Design review of the part built by this model. Coordinates are the model's own, in mm. Face numbers are marked on the shaded views. A direction names the side the tool comes from. Coordinates: 2 decimals unless noted, no trailing zeros. Write each loop counter-clockwise with the first axis right and the second up, starting at its lowest first coordinate (ties: lowest second). Pieces come first, ordered by that corner, then holes. Notation, with made-up numbers: (44.25, -5.75) - (80.25, -5.75) arc R25 cw to (80.25, 9.25) - close; hole circle Ø6 at (43, -6). An arc over 180 degrees is marked (long way). Answer as a JSON object with one key per item and string values.
```python
from build123d import *

# Parameters (mm, degrees)
BOSS_EXTRUDE1_DEPTH = 2.032


with BuildPart() as part:
    # Sketch1 → Boss-Extrude1 (new body)
    with BuildSketch(Plane.XY):
        Polygon((2.794, 7.39775), (-2.794, 7.39775), (-5.5245, 4.66725), (-5.5245, -4.66725), (5.5245, -4.66725), (5.5245, 4.66725), align=None)
        with BuildLine():
            ThreePointArc((1.75976362, 1.016), (0, -2.032), (-1.75976362, 1.016))
            Line((-1.75976362, 1.016), (1.75976362, 1.016))
        make_face(mode=Mode.SUBTRACT)
    extrude(amount=BOSS_EXTRUDE1_DEPTH)


solid = part.part
```
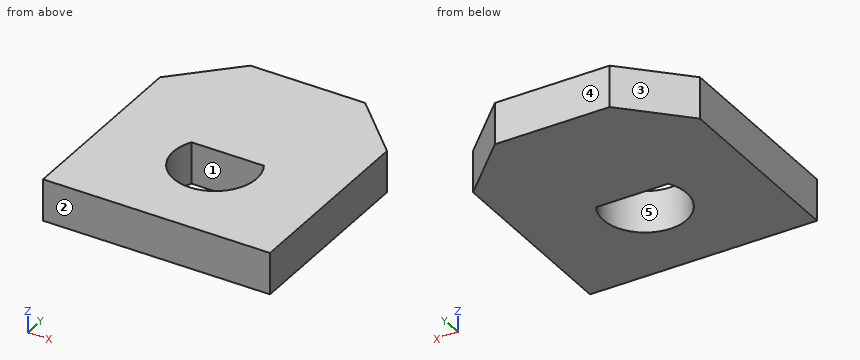
(1) Take a section at D-D, the plane y = 6.25. Write out the cut boundary in (x, z).
Solved:
{"outline": "(-3.94, 0) - (3.94, 0) - (3.94, 2.03) - (-3.94, 2.03) - close"}
(2) Take a section at A-A, the plane z = 1.6. Write out the cut boundary in (x, y).
Solved:
{"outline": "(-5.52, -4.67) - (5.52, -4.67) - (5.52, 4.67) - (2.79, 7.4) - (-2.79, 7.4) - (-5.52, 4.67) - close; hole (-1.76, 1.02) arc R2.03 ccw (long way) to (1.76, 1.02) - close"}
(3) Take a section at B-B, the plane y = 0. Write out the cut boundary in (x, z), and give its area (3 significant figures).
Solved:
{"outline": "(-5.52, 0) - (-2.03, 0) - (-2.03, 2.03) - (-5.52, 2.03) - close; (2.03, 0) - (5.52, 0) - (5.52, 2.03) - (2.03, 2.03) - close", "area": "14.2 mm^2"}
(4) The part is to be moulded in two halves that separate along X. For the marked faces 3, 4 and 5, say which applies: pulls with the +X half, pulls with the -X half, needs draft (parallel to the pull), parting line crosses it, or undercut.
Solved:
{"face 3": "pulls with the -X half", "face 4": "needs draft", "face 5": "undercut"}
(5) Take a section at C-C, the plane x = 0. Write out the cut boundary in (y, z), and give its area (3 significant figures).
Solved:
{"outline": "(-4.67, 0) - (-2.03, 0) - (-2.03, 2.03) - (-4.67, 2.03) - close; (1.02, 0) - (7.4, 0) - (7.4, 2.03) - (1.02, 2.03) - close", "area": "18.3 mm^2"}
(6) Tool access review of the marked faces 1 and 2: name each direction out of +Z, -Z, +X, -X, +Y, -Y from which nothing blocks a thin tool from reaching the whole face with its end or side.
Solved:
{"face 1": "+Z, -Z", "face 2": "+Z, -Z, +X, -X, -Y"}
(7) To check wall thickness, follow line 1 (X direction, y = 0, z = 0.9); line 2 (Y direction, x = -1.5, z = 0.3); line 3 (X direction, y = -1, z = 1.35). State the ranges of each line that lie inside material, in increasing order. Write a range as from..to.
Solved:
{"line 1": "x = -5.52..-2.03, 2.03..5.52", "line 2": "y = -4.67..-1.37, 1.02..7.4", "line 3": "x = -5.52..-1.77, 1.77..5.52"}
